Autodesk Inventor part; units mm, degrees
ref_plane "YZ Plane" through (0, 0, 0) normal (1, 0, 0) x (0, 1, 0)
ref_plane "XZ Plane" through (0, 0, 0) normal (0, 1, 0) x (-1, 0, 0)
ref_plane "XY Plane" through (0, 0, 0) normal (0, 0, 1) x (1, 0, 0)
sketch "Sketch1" plane through (0, 0, 0) normal (0, 1, 0) x (-1, 0, 0)
  line L0 (35, 0) -> (-35, 0)
  circle A0 centre (-35, 0) radius 7.5
  circle A1 centre (35, 0) radius 7.5
  circle A2 centre (35, 0) radius 50
  circle A3 centre (-35, 0) radius 50
  line L1 (35, -50) -> (-35, -50)
  line L2 (0, -50) -> (0, -35.5)
  line L3 (15.5, -35.5) -> (-15.5, -35.5)
  line L4 (15.5, -35.5) -> (-15.5, -35.5)
  line L5 (-15.5, -35.5) -> (-15.5, -4.5)
  line L6 (-15.5, -4.5) -> (15.5, -4.5)
  line L7 (15.5, -4.5) -> (15.5, -35.5)
  circle A4 centre (15.5, -35.5) radius 1.8
  circle A5 centre (-15.5, -35.5) radius 1.8
  circle A6 centre (-15.5, -4.5) radius 1.8
  circle A7 centre (15.5, -4.5) radius 1.8
  line L8 (15.5, -35.5) -> (-15.5, -4.5)
  line L9 (-15.5, -4.5) -> (-15.5, -35.5)
  line L10 (-15.5, -35.5) -> (15.5, -4.5)
  circle A8 centre (0, -20) radius 11
  line L11 (0, 0) -> (0, 50)
  circle A9 centre (0, 50) radius 10
  line L12 (47.1461, 48.5023) -> (2.4292, 59.7005)
  line L13 (-2.4292, 59.7005) -> (-47.1461, 48.5023)
  point P0 (0, 35.7071)
  dimension "d0" = 70
  dimension "d1" = 15
  dimension "d2" = 15
  dimension "d3" = 100
  dimension "d4" = 100
  dimension "d5" = 14.5
  dimension "d6" = 31
  dimension "d7" = 31
  dimension "d8" = 3.6
  dimension "d9" = 3.6
  dimension "d10" = 3.6
  dimension "d11" = 3.6
  dimension "d14" = 22
  dimension "d15" = 50
  dimension "d16" = 20
extrude "Extrusion1" add sketch "Sketch1" along normal blind 2 contours A3 A7 L6 A6 A2 L0 | L0 L11 A3 | A3 A2 L3 A4 L7 A7 | L0 A2 L11 | L11 A9 L12 A2 | A2 A6 L5 A5 L3 A3 | A3 L13 A9 L11 | A9 | A7 L10 A8 L8 A6 L6 | A3 L2 L1 | L7 A4 L8 A8 A3 A7 | A7 A3 A8 L10 | A6 A2 A8 L10 A5 L5 | L1 L2 A2 | L2 L3 A3 | A2 L3 L2 | L8 A8 A2 A6 | L3 A5 L10 A8 A2 | A2 A8 A3 L3 | A3 A8 L8 A4 L3
properties part number "Extruder Frame"
Source: CAD feature listing. Evaluate the final solid. Frame: model axes, mm. Round coordinates to 2 decimals unless told otherwise and drop trailing zeros. Loops run counter-clockwise (first coordinate to the right, second up) from the corner with the lowest first, then second, coordinate; pieces in that order, holes last.
Q1. Section C-C, the plane y = 0.85. Return loops of the section in (x, z).
Q2. Section A-A, the plane z = 0. Return loops of the section in (x, y).
Q3. Ray query, line 1 (Z direction, x = 15.5, y = 1.5); line 2 (X direction, y = 1.2, z = -4); line 3 (X direction, y = 1.25, z = -2). Return the intervals inside material, ascending.
Q4. Section D-D, the plane z = -16. Return loops of the section in (x, y).
Q5. First-contact query: P1, Ø13.5, axis at x = 35, z = 0, coming from the +Y side; P2, Ø1, axis at y = 1.5, z = 28, coming from the +X side. Flat tips, straight axial feed; report the tip coordinate or a pass-through.
Q6. Mould query, pull axis Z, two halves, no side actions, for faces 1 (the face through (24.47, 0.99, 54.18)), 2 (the face through (1, 2, 6)), 3 (the face through (-17.217, 0.986, -36.041)). Classes: pulls with the +Z half, pulls with the -Z half, needs draft (parallel to the pull), parting line crosses it, or undercut.
Q7. Section B-B, the plane x = 0. Return loops of the section in (y, z), plus the area to 3 significant figures.
Solutions:
1. outline: (-47.15, 48.5) arc R50 ccw to (-35, -50) - (35, -50) arc R50 ccw to (47.15, 48.5) - (2.43, 59.7) arc R10 ccw to (-2.43, 59.7) - close; hole circle Ø15 at (-35, 0); hole circle Ø3.6 at (-15.5, -35.5); hole circle Ø3.6 at (-15.5, -4.5); hole circle Ø22 at (0, -20); hole circle Ø3.6 at (15.5, -35.5); hole circle Ø3.6 at (15.5, -4.5); hole circle Ø15 at (35, 0)
2. outline: (-85, 0) - (-42.5, 0) - (-42.5, 2) - (-85, 2) - close; (-27.5, 0) - (27.5, 0) - (27.5, 2) - (-27.5, 2) - close; (42.5, 0) - (85, 0) - (85, 2) - (42.5, 2) - close
3. line 1: z = -50 to -37.3, -33.7 to -6.3, -2.7 to 56.43
3. line 2: x = -84.84 to -41.34, -28.66 to -17.23, -13.77 to 13.77, 17.23 to 28.66, 41.34 to 84.84
3. line 3: x = -84.96 to -42.23, -27.77 to 27.77, 42.23 to 84.96
4. outline: (-82.37, 0) - (-10.25, 0) - (-10.25, 2) - (-82.37, 2) - close; (10.25, 0) - (82.37, 0) - (82.37, 2) - (10.25, 2) - close
5. P1: passes through
5. P2: stops at x = 76.76
6. face 1: pulls with the +Z half
6. face 2: needs draft
6. face 3: undercut
7. outline: (0, -50) - (2, -50) - (2, -31) - (0, -31) - close; (0, -9) - (2, -9) - (2, 60) - (0, 60) - close
7. area: 176 mm2
